CAD build for the part. Positions are in the model's coordinates, mm. Give positions to 0.01 mm unless a question says otherwise; leave off trailing zeros. Loops run counter-clockwise (first coordinate to the right, second up) from the corner with the lowest first, then second, coordinate; pieces in that order, holes last.
```python
from build123d import *

# Parameters (mm, degrees)
F0_W     = 2.2499504322
F0_H     = 1.7434554408
F1_DEPTH = 1.1348915286
F3_DEPTH = 1.8342579715
F4_DEPTH = 33.0712201539


# Not quite as in the source:
# - the program builds the solid bodies; features that only make, move or delete a surface that nothing else refers to are left out


with BuildPart() as f1:
    # F0 (on Top) → F1 (new body)
    with BuildSketch(Plane.XY):
        Polygon((6.35, 1.2873262627), (-6.35, 1.2873262627), (-6.35, 0.6436631313), (-8.2549656289, 0.6436631313), (-8.2549656289, 0), (-6.35, 0), (-6.35, -1.2873262627), (6.35, -1.2873262627), (6.35, 0), (8.2549656289, 0), (8.2549656289, 0.6436631313), (6.35, 0.6436631313), align=None)
        with Locations((3.175, 0)):
            Rectangle(F0_W, F0_H, mode=Mode.SUBTRACT)
        with Locations((-3.175, 0)):
            Rectangle(F0_W, F0_H, mode=Mode.SUBTRACT)
    extrude(amount=F1_DEPTH)

    # F0 (on Top) → F3 (join)
    with BuildSketch(Plane.XY):
        with Locations((-3.175, 0)):
            Rectangle(F0_W, F0_H)
    extrude(amount=F3_DEPTH)

    # F0 (on Top) → F4 (join)
    with BuildSketch(Plane.XY):
        Polygon((6.35, 1.2873262627), (-6.35, 1.2873262627), (-6.35, 0.6436631313), (-8.2549656289, 0.6436631313), (-8.2549656289, 0), (-6.35, 0), (-6.35, -1.2873262627), (6.35, -1.2873262627), (6.35, 0), (8.2549656289, 0), (8.2549656289, 0.6436631313), (6.35, 0.6436631313), align=None)
        with Locations((3.175, 0)):
            Rectangle(F0_W, F0_H, mode=Mode.SUBTRACT)
        with Locations((-3.175, 0)):
            Rectangle(F0_W, F0_H, mode=Mode.SUBTRACT)
    extrude(amount=F4_DEPTH)


solid = f1.part
```
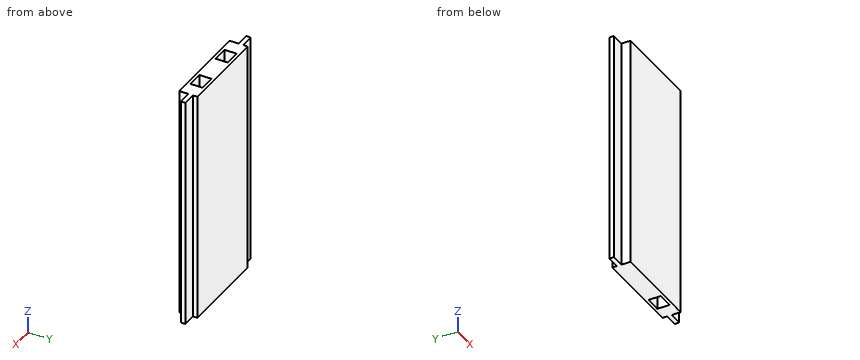
1. Saw through at C-C, the plane x = -3.5. List the corners of the cut face in (y, z).
Responses:
outline: (-1.29, 0) - (1.29, 0) - (1.29, 33.07) - (0.87, 33.07) - (0.87, 1.83) - (-0.87, 1.83) - (-0.87, 33.07) - (-1.29, 33.07) - close
2. Drop flat-ended pins along their axis: pin 1 (0.6 mm diameter, centred on x = 7, z = 12, fed in from +Y); pin 2 (0.6 mm diameter, centred on x = 7, z = 17, fed in from -Y). Give the stop position or say it passes through.
Responses:
pin 1: stops at y = 0.64
pin 2: stops at y = 0
3. Saw through at D-D, the plane x = -6.75. List the corners of the cut face in (y, z), and give its area (3 significant figures).
Responses:
outline: (0, 0) - (0.64, 0) - (0.64, 33.07) - (0, 33.07) - close
area: 21.3 mm2
4. Saw through at B-B, the plane z = 16.5. List the corners of the cut face in (x, y).
Responses:
outline: (-8.25, 0) - (-6.35, 0) - (-6.35, -1.29) - (6.35, -1.29) - (6.35, 0) - (8.25, 0) - (8.25, 0.64) - (6.35, 0.64) - (6.35, 1.29) - (-6.35, 1.29) - (-6.35, 0.64) - (-8.25, 0.64) - close; hole (-4.3, -0.87) - (-2.05, -0.87) - (-2.05, 0.87) - (-4.3, 0.87) - close; hole (2.05, -0.87) - (4.3, -0.87) - (4.3, 0.87) - (2.05, 0.87) - close
5. Saw through at A-A, the plane y = -0.45. List the corners of the cut face in (x, z).
Responses:
outline: (-6.35, 0) - (2.05, 0) - (2.05, 33.07) - (-2.05, 33.07) - (-2.05, 1.83) - (-4.3, 1.83) - (-4.3, 33.07) - (-6.35, 33.07) - close; (4.3, 0) - (6.35, 0) - (6.35, 33.07) - (4.3, 33.07) - close
6. Probe line 1 along X through (y, z) = (0.05, 11.5); line 2 along X through (y, z) = (0.8, 17.5); line 3 along Y through (x, z) = (-3, 17). List the from-to ranges inside material, lowest first.
Responses:
line 1: x = -8.25 to -4.3, -2.05 to 2.05, 4.3 to 8.25
line 2: x = -6.35 to -4.3, -2.05 to 2.05, 4.3 to 6.35
line 3: y = -1.29 to -0.87, 0.87 to 1.29
